Source: CAD feature listing. Evaluate the final solid. Frame: model axes, mm. A direction names the side the tool comes from. Round coordinates to 2 decimals unless told otherwise and drop trailing zeros. Loops run counter-clockwise (first coordinate to the right, second up) from the corner with the lowest first, then second, coordinate; pieces in that order, holes last. Notation, with made-up numbers: (27, -6.75) - (45, -6.75) arc R19 cw to (45, 27.25) - close; hole circle Ø8 at (23.25, 72.25). An arc over 180 degrees is marked (long way). One line per question, with ' | ' between items. Start each with the question number.
1. Cut plane B-B (z = 4.5). Return loops of the section in (x, y).
2. Cut plane A-A (x = 11.5). Return loops of the section in (y, z), then the cut area to 3 significant figures.
3. Cut plane C-C (y = 0.85). Return loops of the section in (x, z).
4. Mould query, pull axis X, two halves, no side actions, for faces 3 (the flat face through (0, 1, -40)), 4 (the flat face through (0, 1, 12.5)), 5 (the cylindrical face through (36.99, 0.86, -37.15)). Classes: pulls with the +X half, pulls with the -X half, needs draft (parallel to the pull), parting line crosses it, or undercut.
5. Access query for faces 1 (the flat face through (-18, 1, 0)), 2 (the flat face through (40, 1, 0)). Directions: +Z, -Z, +X, -X, +Y, -Y. A direction counts if a zero-diameter tool reaches every point of the face in a straight line with its end or side. Return the directions, or none.
6. Ray query, line 1 (Z direction, x = -5.5, y = 0.1); line 2 (X direction, y = 0.65, z = -9); line 3 (Z direction, x = 35.5, y = 0.45). Return the intervals inside material, ascending.
```python
from build123d import *

# Parameters (mm, degrees)
ESQUISSE1_W        = 80
ESQUISSE1_H        = 80
ESQUISSE1_W_2      = 36
ESQUISSE1_H_2      = 25
BOSS_EXTRU_1_DEPTH = 1.7
CONG_1_R           = 10


with BuildPart() as part:
    # Esquisse1 → Boss.-Extru.1 (new body)
    with BuildSketch(Plane(origin=(0, 0, 0), x_dir=(1, 0, 0), z_dir=(0, 1, 0))):
        Rectangle(ESQUISSE1_W, ESQUISSE1_H)
        Rectangle(ESQUISSE1_W_2, ESQUISSE1_H_2, mode=Mode.SUBTRACT)
    extrude(amount=BOSS_EXTRU_1_DEPTH)

    # Congé1
    cong_1_edges = [part.edges().sort_by_distance(p)[0] for p in [
        (-40, 0.85, -40),
        (-40, 0.85, 40),
        (40, 0.85, 40),
        (40, 0.85, -40),
    ]]
    fillet(cong_1_edges, radius=CONG_1_R)


solid = part.part
```
Answers follow:
1) outline: (-40, 0) - (-18, 0) - (-18, 1.7) - (-40, 1.7) - close; (18, 0) - (40, 0) - (40, 1.7) - (18, 1.7) - close
2) outline: (0, -40) - (1.7, -40) - (1.7, -12.5) - (0, -12.5) - close; (0, 12.5) - (1.7, 12.5) - (1.7, 40) - (0, 40) - close | area: 93.5 mm2
3) outline: (-40, -30) arc R10 ccw to (-30, -40) - (30, -40) arc R10 ccw to (40, -30) - (40, 30) arc R10 ccw to (30, 40) - (-30, 40) arc R10 ccw to (-40, 30) - close; hole (-18, -12.5) - (18, -12.5) - (18, 12.5) - (-18, 12.5) - close
4) face 3: needs draft | face 4: undercut | face 5: pulls with the +X half
5) face 1: +Y, -Y | face 2: +Z, -Z, +X, +Y, -Y
6) line 1: z = -40 to -12.5, 12.5 to 40 | line 2: x = -40 to -18, 18 to 40 | line 3: z = -38.35 to 38.35
